Autodesk Inventor part; units mm, degrees
ref_plane "YZ Plane" through (0, 0, 0) normal (1, 0, 0) x (0, 1, 0)
ref_plane "XZ Plane" through (0, 0, 0) normal (0, 1, 0) x (-1, 0, 0)
ref_plane "XY Plane" through (0, 0, 0) normal (0, 0, 1) x (1, 0, 0)
sketch "Sketch1" plane through (0, 0, 0) normal (0, 0, 1) x (1, 0, 0)
  arc A0 (5, -27.0416) -> (5, 27.0416) centre (0, 0) ccw
  line L0 (9.25, 0) -> (0.933, 0)
  line L1 (5, -27.5) -> (5, -13.7954)
  arc A1 (5, -13.7954) -> (5, 13.7954) centre (-4.5, 0) ccw
  arc A2 (5, -27.0416) -> (5, 27.0416) centre (0, 0) ccw
  line L2 (5, 27.5) -> (5, 13.7954)
  line L3 (5, -13.7954) -> (5, -27.5)
  point P0 (-3.7885, 24.6247)
extrude "Extrusion1" add sketch "Sketch1" along normal blind 7.5
sketch "Sketch3" plane through (5, -27.0416, 0) normal (-1, 0, 0) x (0, 0, 1)
  line L0 (0, 6.9167) -> (7.5, 6.9167)
  line L1 (0, 0) -> (0, 6.9167)
  line L2 (0, 6.9167) -> (7.5, 6.9167)
  line L3 (7.5, 26.7893) -> (7.5, 0)
  line L4 (7.5, 6.9167) -> (7.5, 0)
  line L5 (7.5, 0) -> (0, 0)
  line L6 (7.5, 0) -> (0, 0)
  circle A0 centre (3.75, 3.963) radius 1
  line L7 (0, 0) -> (0, 53.5786)
  line L8 (0, 53.5786) -> (0, 0)
  line L9 (0, 26.7893) -> (7.5, 26.7893)
  circle A1 centre (3.75, 50.6249) radius 1
  line L10 (0, 53.5786) -> (7.5, 53.5786)
  line L11 (7.5, 53.5786) -> (7.5, 0)
  line L12 (7.5, 54.0833) -> (0.9403, 54.0833)
  line L13 (0, 54.0833) -> (7.5, 54.0833)
  circle A2 centre (3.75, 3.963) radius 2
  circle A3 centre (3.75, 50.6249) radius 2
  point P0 (0, 27.0416)
  point P1 (280.32, 51.414)
  dimension "d7" = 2
  dimension "d10" = 4
  dimension "d11" = 4
extrude "Extrusion3" cut sketch "Sketch3" against normal blind 25.4 contours A0 | A1
extrude "Extrusion4" cut sketch "Sketch3" against normal blind 17.9375 contours A2 | A3
scale "Scale1" factors (0.5, 0.5, 0.5) then translate (2.5, -6.8977, 3.75) bodies 1
properties part number "Contrapeso2"
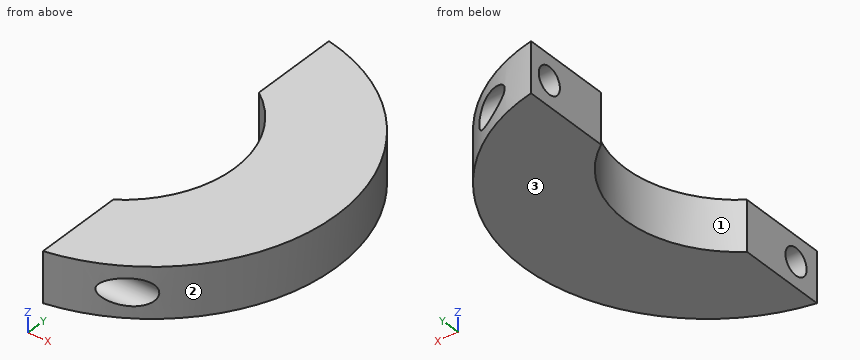
Geometry: final body of the model. Coordinates: model frame, mm. Face numbers are marked on the shaded views. Coordinates: 2 decimals unless noted, no trailing zeros. Write each loop counter-clockwise with the first axis right and the second up, starting at its lowest first coordinate (ties: lowest second). Pieces come first, ordered by that corner, then holes. Notation, with made-up numbers: M 87,61.5 L 145,61.5 A23 ccw 145,95.5 Z; hole C 21.25,-21 d1. An arc over 180 degrees is marked long. Answer as CSV lines item,"result". Start each with the question number.
Q1. Cut plane D-D on y = -5.5. Return the cut outline in (x, z).
Q2. Cut plane B-B on z = 6.1. Count the separate pieces of the cut face and the enclosed holes in it, then the cut area to 3 significant figures.
Q3. Line query: line 1 (Y direction, x = 8, z = 6.05); line 2 (Y direction, x = 7.25, z = 5.95); line 3 (Z direction, x = 8.25, y = -19). Output: solid intervals per line, ascending. Write a range as from..to.
Q4. Cut plane A-A on x = 8. Return the cut outline in (y, z) (3 decimals), then the cut area to 3 significant figures.
Q5. Mould query, pull axis Y, two halves, no side actions, for the marked faces 1, 2 and 3. Classes: released by +Y, released by -Y, zero draft, split by the parting line, or undercut.
Q6. Cut plane C-C on x = 6.5. Return the cut outline in (y, z) (3 decimals).
Q7. Pin query (flat end, axial travel): P1, Ø1.6, axis at y = 4.89, z = 5.62, coming from the -X side. Return the tip coordinate at first contact, or that it passes through.
Findings below:
1,outline,"M 8.51,3.75 L 16.18,3.75 L 16.18,7.5 L 8.51,7.5 Z"
2,separate pieces,"3"
2,enclosed holes,"0"
2,area,"177 mm2"
3,line 1,"y = -19.5..-19.34, -17.53..-10.07, -3.72..3.99"
3,line 2,"y = -19.8..-19.38, -17.49..-11.5, -2.3..3.95, 5.84..6.01"
3,line 3,"z = 3.75..4.8, 6.45..7.5"
4,outline,"M -19.5,3.75 L -10.072,3.75 L -10.072,7.5 L -19.5,7.5 Z; M -3.723,3.75 L 5.704,3.75 L 5.704,5.039 A1 cw long 5.704,6.211 L 5.704,7.5 L -3.723,7.5 Z; hole C -18.437,5.625 d2"
4,area,"64.6 mm2"
5,face 1,"undercut"
5,face 2,"split by the parting line"
5,face 3,"zero draft"
6,outline,"M -20.053,3.75 L -12.472,3.75 L -12.472,7.5 L -20.053,7.5 Z; M -1.323,3.75 L 6.258,3.75 L 6.258,7.5 L -1.323,7.5 Z; hole C -18.437,5.625 d2; hole C 4.894,5.625 d2"
7,P1,"passes through"
